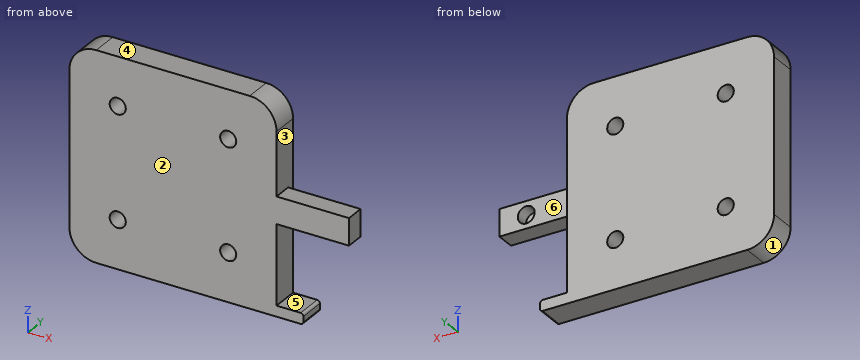
```python
from build123d import *

# Parameters (mm, degrees)
CROQUIS1_W              = 77.15
CROQUIS1_H              = 77.15
CROQUIS1_R              = 3
SALIENTE_EXTRUIR1_DEPTH = 10
REDONDEO1_R             = 10
SALIENTE_EXTRUIR2_DEPTH = 30
CORTAR_EXTRUIR1_START   = -3
CROQUIS3_R              = 3.15
CORTAR_EXTRUIR1_DEPTH   = 5
CORTAR_EXTRUIR2_START   = -3
CROQUIS4_W              = 3
CROQUIS4_H              = 10
CORTAR_EXTRUIR2_DEPTH   = 43
CROQUIS5_W              = 4
CROQUIS5_H              = 10
SALIENTE_EXTRUIR3_DEPTH = 10
REDONDEO2_R             = 1


with BuildPart() as part:
    # Croquis1 → Saliente-Extruir1 (new body)
    with BuildSketch(Plane(origin=(0, 0, 0), x_dir=(1, 0, 0), z_dir=(0, 1, 0))):
        Rectangle(CROQUIS1_W, CROQUIS1_H)
        with Locations(Location((-20.575, -20.575, 0), (0, 0, 270))):
            Circle(CROQUIS1_R, mode=Mode.SUBTRACT)
        with Locations(Location((-20.575, 20.575, 0), (0, 0, 270))):
            Circle(CROQUIS1_R, mode=Mode.SUBTRACT)
        with Locations(Location((20.575, 20.575, 0), (0, 0, 270))):
            Circle(CROQUIS1_R, mode=Mode.SUBTRACT)
        with Locations(Location((20.575, -20.575, 0), (0, 0, 270))):
            Circle(CROQUIS1_R, mode=Mode.SUBTRACT)
    extrude(amount=SALIENTE_EXTRUIR1_DEPTH)

    # Redondeo1
    redondeo1_edges = [part.edges().sort_by_distance(p)[0] for p in [
        (-38.575, 5, 38.575),
        (-38.575, 5, -38.575),
        (38.575, 5, 38.575),
    ]]
    fillet(redondeo1_edges, radius=REDONDEO1_R)

    # Croquis2 → Saliente-Extruir2 (add)
    with BuildSketch(Plane(origin=(38.575, 0, 0), x_dir=(0, 0, -1), z_dir=(1, 0, 0))):
        Polygon((5, 0), (0, 0), (-5, 0), (-5, 7), (5, 7), align=None)
    extrude(amount=SALIENTE_EXTRUIR2_DEPTH)

    # Croquis3 → Cortar-Extruir1 (cut)
    with BuildSketch(Plane(origin=(0, 10, 0), x_dir=(1, 0, 0), z_dir=(0, 1, 0)).offset(CORTAR_EXTRUIR1_START)):
        with Locations(Location((55.575, 0, 0), (0, 0, 90))):
            Circle(CROQUIS3_R)
    extrude(amount=-CORTAR_EXTRUIR1_DEPTH, mode=Mode.SUBTRACT)

    # Croquis4 → Cortar-Extruir2 (cut)
    with BuildSketch(Plane(origin=(0, 10, 0), x_dir=(1, 0, 0), z_dir=(0, 1, 0)).offset(CORTAR_EXTRUIR2_START)):
        with Locations((67.075, 0)):
            Rectangle(CROQUIS4_W, CROQUIS4_H)
    extrude(amount=-CORTAR_EXTRUIR2_DEPTH, mode=Mode.SUBTRACT)

    # Croquis5 → Saliente-Extruir3 (add)
    with BuildSketch(Plane(origin=(38.575, 0, 0), x_dir=(0, 0, -1), z_dir=(1, 0, 0))):
        with Locations((36.575, 5)):
            Rectangle(CROQUIS5_W, CROQUIS5_H)
    extrude(amount=SALIENTE_EXTRUIR3_DEPTH)

    # Redondeo2
    redondeo2_edges = [part.edges().sort_by_distance(p)[0] for p in [
        (48.575, 5, -38.575),
        (48.575, 5, -34.575),
    ]]
    fillet(redondeo2_edges, radius=REDONDEO2_R)


solid = part.part
```
For this review, take the finished solid that the model builds, in its own axes (mm). Face numbers are marked on the shaded views. A direction names the side the tool comes from. Round coordinates to 2 decimals unless told otherwise and drop trailing zeros. Write each loop counter-clockwise with the first axis right and the second up, starting at its lowest first coordinate (ties: lowest second). Pieces come first, ordered by that corner, then holes. Notation, with made-up numbers: (-32, 35) - (-8, 35) arc R21 cw to (-8, 69) - close; hole circle Ø1 at (-3, -11.5). An arc over 180 degrees is marked (long way). Put each result on its own line as item: value.
Q1. We need section B-B (y = 5.5). Give the boundary of the cut face in (x, z) (3 decimals), and give its area (3 significant figures).
Solved:
outline: (-38.575, -28.575) arc R10 ccw to (-28.575, -38.575) - (47.575, -38.575) arc R1 ccw to (48.575, -37.575) - (48.575, -35.575) arc R1 ccw to (47.575, -34.575) - (38.575, -34.575) - (38.575, -5) - (65.575, -5) - (65.575, 5) - (38.575, 5) - (38.575, 28.575) arc R10 ccw to (28.575, 38.575) - (-28.575, 38.575) arc R10 ccw to (-38.575, 28.575) - close; hole circle Ø6 at (-20.575, -20.575); hole circle Ø6 at (-20.575, 20.575); hole circle Ø6 at (20.575, -20.575); hole circle Ø6 at (20.575, 20.575); hole circle Ø6.3 at (55.575, 0)
area: 6,050 mm2
Q2. We need section A-A (z = -22.5). Give the boundary of the cut face in (x, y) (3 decimals).
Solved:
outline: (-38.575, 0) - (-22.876, 0) - (-22.876, 10) - (-38.575, 10) - close; (-18.274, 0) - (18.274, 0) - (18.274, 10) - (-18.274, 10) - close; (22.876, 0) - (38.575, 0) - (38.575, 10) - (22.876, 10) - close
Q3. Wall thickness on probe 1 along X at (y, z) = (4.5, 18.5) (3 decimals); probe 2 along Z at (x, y) = (-19.5, 8.5) (3 decimals); probe 3 along Z at (x, y) = (46, 4.25) (3 decimals): over which ranges is each line inside the solid? List them lowest first.
Solved:
probe 1: x = -38.575 to -22.742, -18.408 to 18.408, 22.742 to 38.575
probe 2: z = -38.575 to -23.376, -17.774 to 17.774, 23.376 to 38.575
probe 3: z = -38.575 to -34.575, -5 to 5
Q4. We need section C-C (z = 0). Give the boundary of the cut face in (x, y) (3 decimals), and give its area (3 significant figures).
Solved:
outline: (-38.575, 0) - (65.575, 0) - (65.575, 7) - (58.725, 7) - (58.725, 2) - (52.425, 2) - (52.425, 7) - (38.575, 7) - (38.575, 10) - (-38.575, 10) - close
area: 929 mm2
Q5. Mouldability with a two-part tool opening along Z and no side actions: class the marked faces 1, 2 and 3 as released by +Z, released by -Z, zero draft, split by the parting line, or undercut.
Solved:
face 1: released by -Z
face 2: zero draft
face 3: undercut
Q6. Machinability: for the marked faces 4, 5 and 6, which of the approach directions +Z, -Z, +X, -X, +Y, -Y give a long, thin tool a straight path to every point of the face, cutting with its end or side? Answer none if there is none.
Solved:
face 4: +Z, +X, -X, +Y, -Y
face 5: +X, +Y, -Y
face 6: +Z, +X, +Y
Q7. Insertion check: pin 1 Ø2.5 at (x, y) = (45.5, 5) entering from +Z; pin 2 Ø6 at (y, z) = (1.5, 24) entering from +X (3 decimals); pin 3 Ø1 at (y, z) = (7, -36.5) entering from +X (3 decimals); pin 4 Ø8 at (x, z) = (20.575, 20.575) entering from -Y. Each pin has a flat end and moves straight along its axis. Give the tip position at first contact, or say it passes through.
Solved:
pin 1: stops at z = 5
pin 2: stops at x = 38.575
pin 3: stops at x = 48.575
pin 4: stops at y = 0
Q8. We need section D-D (z = -30.5). Give the boundary of the cut face in (x, y) (3 decimals).
Solved:
outline: (-38.388, 0) - (38.575, 0) - (38.575, 10) - (-38.388, 10) - close
